Here's how the part is built. I have some questions about the finished solid (model axes, mm). Face numbers are marked on the shaded views. A direction names the side the tool comes from. Coordinates: 2 decimals unless noted, no trailing zeros. Order: outer loops, then holes, each group sorted by start corner. A loop starts at its lowest first (then second) coordinate and runs counter-clockwise, first axis right, second up. Notation, with made-up numbers: (-13, 54.25) - (44, 54.25) arc R31 cw to (44, 88.25) - close; hole circle Ø4 at (56.25, 28.5). An arc over 180 degrees is marked (long way). Use CSV: the item, a comma, the result in double quotes. Start each with the question number.
from build123d import *

# Parameters (mm, degrees)
SKETCH1_W           = 70
SKETCH1_H           = 20
BOSS_EXTRUDE1_DEPTH = 5
SKETCH2_R           = 10
SKETCH2_R_2         = 6.35
BOSS_EXTRUDE2_DEPTH = 11
SKETCH3_R           = 1.75
CUT_EXTRUDE1_DEPTH  = 44.370496884
FILLET1_R           = 10


with BuildPart() as part:
    # Sketch1 → Boss-Extrude1 (new body)
    with BuildSketch(Plane.XY):
        Rectangle(SKETCH1_W, SKETCH1_H)
    extrude(amount=BOSS_EXTRUDE1_DEPTH)

    # Sketch2 → Boss-Extrude2 (add)
    # profile 1 of 2: a face of its own
    with BuildSketch(Plane.XY.offset(5)):
        with Locations(Location((-25, 0, 0), (0, 0, 180))):
            Circle(SKETCH2_R)
        with Locations((-25, 0)):
            Circle(SKETCH2_R_2, mode=Mode.SUBTRACT)
    # profile 2 of 2: a face of its own
    with BuildSketch(Plane.XY.offset(5)):
        with Locations((25, 0)):
            Circle(SKETCH2_R)
        with Locations((25, 0)):
            Circle(SKETCH2_R_2, mode=Mode.SUBTRACT)
    extrude(amount=BOSS_EXTRUDE2_DEPTH)

    # Sketch3 → Cut-Extrude1 (cut, through all)
    with BuildSketch(Plane(origin=(0, 10, 0), x_dir=(1, 0, 0), z_dir=(0, 1, 0))):
        with Locations(Location((-25, -10.5, 0), (0, 0, 270))):
            Circle(SKETCH3_R)
        with Locations(Location((25, -10.5, 0), (0, 0, 270))):
            Circle(SKETCH3_R)
    extrude(amount=-CUT_EXTRUDE1_DEPTH, mode=Mode.SUBTRACT)

    # Fillet1
    fillet1_edges = [part.edges().sort_by_distance(p)[0] for p in [
        (-35, -10, 2.5),
        (-35, 10, 2.5),
        (35, 10, 2.5),
        (35, -10, 2.5),
    ]]
    fillet(fillet1_edges, radius=FILLET1_R - 0.0001)  # a hair under: the kernel refuses the full size


solid = part.part
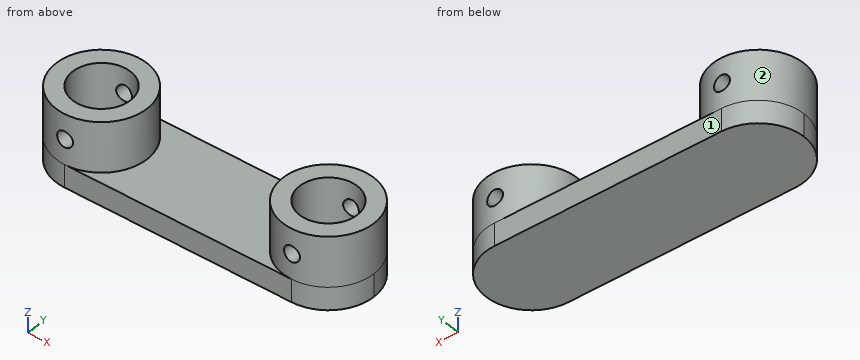
Item 1: Suppose I cut it at A-A on z = 10.5. Write out the boundary of the cut face in (x, y).
Item 2: Suppose I cut it at C-C on x = 18. Write out the boundary of the cut face in (y, z).
Item 3: For pin 1 Ø10 at (x, y) = (13.5, 6.5) entering from +Z; pin 2 Ø3 at (x, z) = (-6, 8) entering from -Y; pin 3 Ø1 at (y, z) = (-6.5, 12) entering from -X; pin 4 Ø4 at (x, y) = (28, 3) entering from +Z, each with a flat end and sliding along its axis, tell me the tip position at first contact or that it passes through.
Item 4: Suppose I cut it at B-B on y = -7.5. State how many separate pieces and enclosed holes the cut face has, then the cut area to 3 significant figures.
Item 5: For the marked faces 1 and 2, which set-ups out of +Z, -Z, +X, -X, +Y, -Y let a thin tool reach every point of the face, with its end or its side?
Item 6: Please list where these lines run through material, in increasing order: line 1 along X through (y, z) = (6.9, 10.5); line 2 along Z through (x, y) = (-25, -7.25); line 3 along X through (y, z) = (-9.15, 10.5). Write a range as from..to.
Here are the results:
1,outline,"(-26.75, -9.85) - (-26.75, -6.1) arc R6.35 cw to (-26.75, 6.1) - (-26.75, 9.85) arc R10 ccw to start; (-23.25, -9.85) arc R10 ccw to (-23.25, 9.85) - (-23.25, 6.1) arc R6.35 cw to (-23.25, -6.1) - close; (23.25, -9.85) - (23.25, -6.1) arc R6.35 cw to (23.25, 6.1) - (23.25, 9.85) arc R10 ccw to start; (26.75, -9.85) arc R10 ccw to (26.75, 9.85) - (26.75, 6.1) arc R6.35 cw to (26.75, -6.1) - close"
2,outline,"(-10, 0) - (10, 0) - (10, 5) - (7.14, 5) - (7.14, 16) - (-7.14, 16) - (-7.14, 5) - (-10, 5) - close"
3,pin 1,"z = 16"
3,pin 2,"through"
3,pin 3,"x = -33"
3,pin 4,"z = 5"
4,separate pieces,"1"
4,enclosed holes,"2"
4,area,"588 mm^2"
5,face 1,"+Z, -Z, +X, -X, +Y"
5,face 2,"+Z"
6,line 1,"-32.24..-26.75, -23.25..-17.76, 17.76..23.25, 26.75..32.24"
6,line 2,"0..8.75, 12.25..16"
6,line 3,"-29.03..-26.75, -23.25..-20.97, 20.97..23.25, 26.75..29.03"
